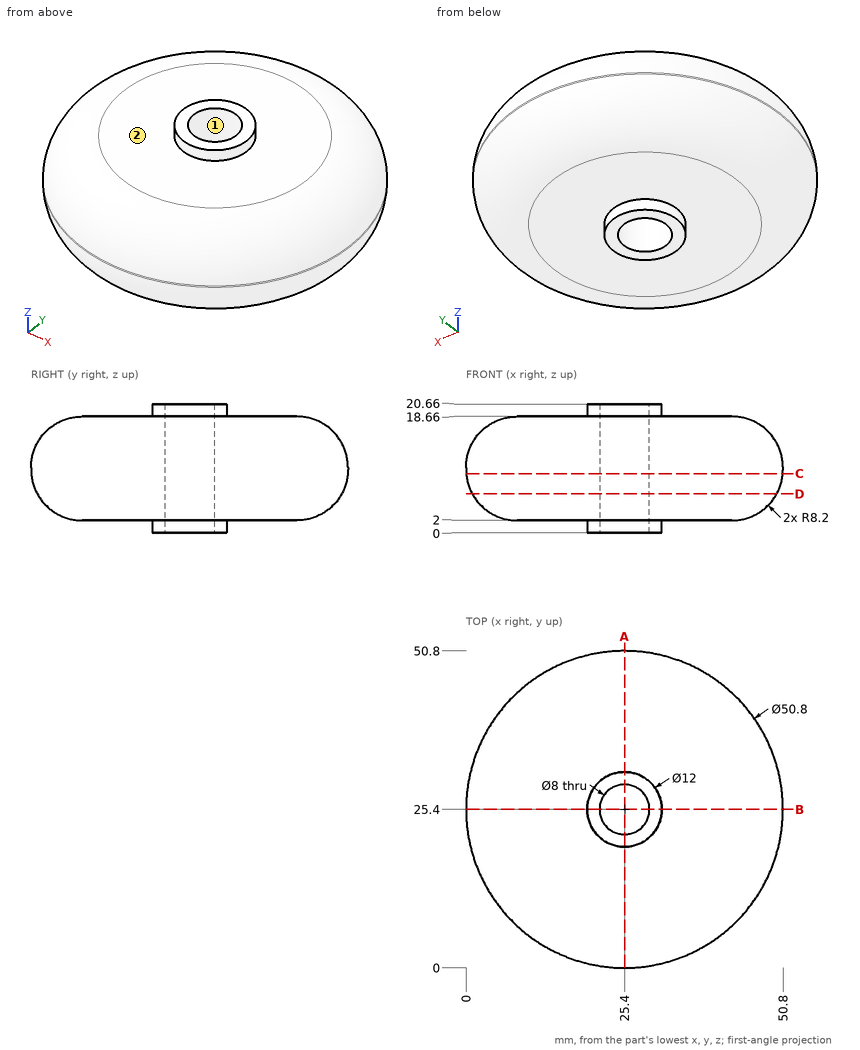
Study the drawing (mm; zero at the part's minimum x, y, z) and answer. Coordinates: 2 decimals unless noted, no trailing zeros. Loops run counter-clockwise (first coordinate to the right, second up) from the corner with the lowest first, then second, coordinate; pieces in that order, holes last. Notation, with made-up numbers: M -1.75,69 L 26.25,69 A25 ccw 26.25,103 Z; hole C -14.5,23 d10. An arc over 180 degrees is marked long. Answer in a Markdown table with one row per item.
1) Find section A-A (x = 25.4). Determine the outline of the cut face in (y, z).
Answers below:
| item | result |
|---|---|
| outline | M 0,10.2 A8.2 ccw 8.2,2 L 19.4,2 L 19.4,0 L 21.4,0 L 21.4,20.66 L 19.4,20.66 L 19.4,18.66 L 8.2,18.66 A8.2 ccw 0,10.46 Z; M 29.4,0 L 31.4,0 L 31.4,2 L 42.6,2 A8.2 ccw 50.8,10.2 L 50.8,10.46 A8.2 ccw 42.6,18.66 L 31.4,18.66 L 31.4,20.66 L 29.4,20.66 Z |
2) Find section C-C (z = 9.5). Determine the outline of the cut face in (x, y).
Answers below:
| item | result |
|---|---|
| outline | C 25.4,25.4 d50.74; hole C 25.4,25.4 d8 |
3) Find the intervals of material crossed by probe 1 along Y at (x, z) = (25.4, 8); probe 2 along Y at (x, z) = (25.4, 8.5); probe 3 along X at (y, z) = (24, 4.25), in increasing order.
Answers below:
| item | result |
|---|---|
| probe 1 | 0.3 to 21.4, 29.4 to 50.5 |
| probe 2 | 0.18 to 21.4, 29.4 to 50.62 |
| probe 3 | 2.6 to 21.65, 29.15 to 48.2 |
4) Given pin 1 (1 mm diameter, centred on x = 37, z = 8, fed in from -Y); pin 2 (2 mm diameter, centred on x = 40, z = 10.5, fed in from -Y); pin 3 (1.5 mm diameter, centred on y = 35.5, z = 15, fed in from +X), each flat-ended and moving along its own axis, determine where each tip first touches the part or whether it passes through.
Answers below:
| item | result |
|---|---|
| pin 1 | y = 2.85 |
| pin 2 | y = 3.95 |
| pin 3 | x = 47.8 |
5) Determine the mould class of the marked faces 1 and 2 for opening direction Y: released by +Y, released by -Y, zero draft, split by the parting line, or undercut.
Answers below:
| item | result |
|---|---|
| face 1 | undercut |
| face 2 | zero draft |
6) Find section D-D (z = 6.25). Determine the outline of the cut face in (x, y), then the cut area to 3 significant figures.
Answers below:
| item | result |
|---|---|
| outline | C 25.4,25.4 d48.77; hole C 25.4,25.4 d8 |
| area | 1,820 mm^2 |
